The model under review builds one solid part; all positions refer to its coordinate system, in mm. A direction names the side the tool comes from. Coordinates: 2 decimals unless noted, no trailing zeros. Order: outer loops, then holes, each group sorted by start corner. A loop starts at its lowest first (then second) coordinate and runs counter-clockwise, first axis right, second up.
```python
from build123d import *

# Parameters (mm, degrees)
SKETCH_1_W                = 60
SKETCH_1_H                = 60
EXTRUDE_1_DEPTH           = 12.6
CHAMFER_1_SIZE            = 2
SKETCH_2_W                = 35
SKETCH_2_H                = 35
EXTRUDE_2_DEPTH           = 0.4
FILLET_1_R                = 2
HOLE_WIZARD_1_D           = 3.4
HOLE_WIZARD_1_CBORE_D     = 6
HOLE_WIZARD_1_CBORE_DEPTH = 5
HOLE_WIZARD_M3_1_D        = 2.5
HOLE_WIZARD_M3_1_DEPTH    = 3.5
HOLE_WIZARD_M3_1_TIP      = 0.751075774


with BuildPart() as part:
    # 草图1 → 凸台-拉伸1 (new body)
    with BuildSketch(Plane.XY):
        Rectangle(SKETCH_1_W, SKETCH_1_H)
    extrude(amount=EXTRUDE_1_DEPTH)

    # 倒角1
    chamfer_1_edges = [part.edges().sort_by_distance(p)[0] for p in [
        (30, -30, 6.3),
        (-30, -30, 6.3),
        (-30, 30, 6.3),
        (30, 30, 6.3),
    ]]
    chamfer(chamfer_1_edges, length=CHAMFER_1_SIZE)

    # 草图2 → 凸台-拉伸2 (add)
    with BuildSketch(Plane.XY.offset(12.6)):
        Rectangle(SKETCH_2_W, SKETCH_2_H)
    extrude(amount=EXTRUDE_2_DEPTH)

    # 圆角1
    fillet_1_edges = [part.edges().sort_by_distance(p)[0] for p in [
        (17.5, -17.5, 12.8),
        (17.5, 17.5, 12.8),
        (-17.5, 17.5, 12.8),
        (-17.5, -17.5, 12.8),
    ]]
    fillet(fillet_1_edges, radius=FILLET_1_R)

    # 孔1 (through all)
    with Locations(Plane(origin=(-25, 25, 12.6), x_dir=(1, 0, 0), z_dir=(0, 0, 1))):
        with Locations((0, 0), (50, 0), (0, -50), (50, -50)):
            CounterBoreHole(HOLE_WIZARD_1_D / 2, HOLE_WIZARD_1_CBORE_D / 2, HOLE_WIZARD_1_CBORE_DEPTH)

    # M3 螺纹孔1
    with Locations(Plane(origin=(-12.5, 12.5, 13), x_dir=(1, 0, 0), z_dir=(0, 0, 1))):
        with Locations((0, 0), (25, 0), (25, -25), (0, -25)):
            Hole(HOLE_WIZARD_M3_1_D / 2, depth=HOLE_WIZARD_M3_1_DEPTH)
            with Locations((0, 0, -(HOLE_WIZARD_M3_1_DEPTH + HOLE_WIZARD_M3_1_TIP / 2))):  # 118° drill point
                Cone(0, HOLE_WIZARD_M3_1_D / 2, HOLE_WIZARD_M3_1_TIP, mode=Mode.SUBTRACT)


solid = part.part
```
(1) Machinability: for faces 4 (the face through (24.086, -23.567, 3.747)), 5 (the face through (12.66, 13.74, 11.23)), which of the approach directions +Z, -Z, +X, -X, +Y, -Y give a long, thin tool a straight path to every point of the face, cutting with its end or side? Answer none if there is none.
A:
face 4: +Z, -Z
face 5: +Z
(2) Wall thickness on probe 1 along Y at (x, z) = (25, 11.45); probe 2 along X at (y, z) = (12.5, 12); probe 3 along Y at (x, z) = (-25, 2): over which ranges is each line inside the solid? List them lowest first.
A:
probe 1: y = -30 to -28, -22 to 22, 28 to 30
probe 2: x = -30 to -13.75, -11.25 to 11.25, 13.75 to 30
probe 3: y = -30 to -26.7, -23.3 to 23.3, 26.7 to 30
(3) We need section C-C, the plane x = -19. Write out the cut boundary in (y, z).
A:
outline: (-30, 0) - (30, 0) - (30, 12.6) - (-30, 12.6) - close
(4) Draft analysis for pull direction Y (two halves, no side actions). For faces 1 (the face through (-29, 29, 6)), 2 (the face through (16.9, -16.93, 12.8)), 3 (the face through (-12.3, -12.58, 8.88)), state which applies: released by +Y, released by -Y, zero draft, split by the parting line, or undercut.
A:
face 1: released by +Y
face 2: released by -Y
face 3: undercut
(5) For pin 1 Ø4 at (x, y) = (25, -25) entering from +Z; pin 2 Ø1.5 at (x, y) = (-9, 22) entering from +Z; pin 3 Ø7 at (x, y) = (-25, 25) entering from -Z; pin 4 Ø2 at (x, y) = (12.5, 12.5) entering from +Z, all flat-tipped, find the tip position at first contact; note any pin that passes through.
A:
pin 1: stops at z = 7.6
pin 2: stops at z = 12.6
pin 3: stops at z = 0
pin 4: stops at z = 9.35
(6) We need section A-A, the plane x = 25. Write out the cut boundary in (y, z).
A:
outline: (-30, 0) - (-26.7, 0) - (-26.7, 7.6) - (-28, 7.6) - (-28, 12.6) - (-30, 12.6) - close; (-23.3, 0) - (23.3, 0) - (23.3, 7.6) - (22, 7.6) - (22, 12.6) - (-22, 12.6) - (-22, 7.6) - (-23.3, 7.6) - close; (26.7, 0) - (30, 0) - (30, 12.6) - (28, 12.6) - (28, 7.6) - (26.7, 7.6) - close
